Here's how the part is built. I have some questions about the finished solid (model axes, mm). A direction names the side the tool comes from. Round coordinates to 2 decimals unless told otherwise and drop trailing zeros. Loops run counter-clockwise (first coordinate to the right, second up) from the corner with the lowest first, then second, coordinate; pieces in that order, holes last. Notation, with made-up numbers: M 66.5,-6 L 113.5,-6 A28 ccw 113.5,18 Z; hole C 51,-27.5 d6. An arc over 180 degrees is marked long. Put each result on its own line as item: value. Start each with the question number.
Autodesk Inventor part; units mm, degrees
ref_plane "YZ Plane" through (0, 0, 0) normal (1, 0, 0) x (0, 1, 0)
ref_plane "XZ Plane" through (0, 0, 0) normal (0, 1, 0) x (-1, 0, 0)
ref_plane "XY Plane" through (0, 0, 0) normal (0, 0, 1) x (1, 0, 0)
sketch "Sketch1" plane through (0, 0, 0) normal (0, 0, 1) x (1, 0, 0)
  line L0 (-75, 75) -> (75, 75)
  line L1 (75, 75) -> (75, -75)
  line L2 (75, -75) -> (-75, -75)
  line L3 (-75, -75) -> (-75, 75)
  line L4 (-75, 75) -> (75, -75) construction
  line L5 (75, 75) -> (-75, -75) construction
  point P0 (0, 0)
  dimension "d0" = 150
  dimension "d1" = 150
extrude "Extrusion1" add sketch "Sketch1" along normal blind 5
sketch "Sketch2" plane through (0, 0, 5) normal (0, 0, 1) x (1, 0, 0)
  line L0 (-65, -65) -> (65, -65)
  line L1 (65, -65) -> (65, 65)
  line L2 (65, 65) -> (-65, 65)
  line L3 (-65, 65) -> (-65, -65)
  line L4 (-65, -65) -> (65, 65) construction
  line L5 (65, -65) -> (-65, 65) construction
  point P0 (0, 0)
  dimension "d4" = 130
  dimension "d5" = 130
extrude "Extrusion2" add sketch "Sketch2" along normal blind 5
chamfer "Chamfer1" distance 2 angle 45 4 edges at (0, -75, 0) (-75, 0, 0) (75, 0, 0) (0, 75, 0)
properties part number "deksel"
1) I'm going to push flat-ended pins straight in: P1, Ø2.5, axis at x = -4.5, z = 6.5, coming from the +Y side; P2, Ø1.5, axis at y = 13.5, z = 8.5, coming from the +X side; P3, Ø2.5, axis at y = 31, z = 6.5, coming from the -X side. Where does each tip first touch, or does it pass through?
2) If I drill on probe 1 along X at (y, z) = (-10, 5.5); probe 2 along Z at (x, y) = (-68, -63.5), over which ranges is the centre line in solid material (lowest first)? Write a range as from..to.
3) On a 3-axis mill with a long thin cutter (end or side, diameter ignored), from which of +Z, -Z, +X, -X, +Y, -Y can I reach the whole of each face in a straight line? I mean faces 1 (the face through (1, 65, 7)), 2 (the face through (65, -1, 7)), 3 (the face through (-65, 1, 7)), 4 (the face through (-1, -65, 7)). Say none if no direction works.
4) Suppose I cut it at A-A (y = 50.5). Write out the boundary of the cut face in (x, z), plus the area to 3 significant figures.
Results are:
1. P1: y = 65
1. P2: x = 65
1. P3: x = -65
2. probe 1: -65..65
2. probe 2: 0..5
3. face 1: +Z, +X, -X, +Y
3. face 2: +Z, +X, +Y, -Y
3. face 3: +Z, -X, +Y, -Y
3. face 4: +Z, +X, -X, -Y
4. outline: M -75,2 L -73,0 L 73,0 L 75,2 L 75,5 L 65,5 L 65,10 L -65,10 L -65,5 L -75,5 Z
4. area: 1,400 mm²
